Check sheet for the modelled part. Datum: model origin and axes. Units: mm. Give positions to 0.01 mm unless a question says otherwise; leave off trailing zeros. Write each loop counter-clockwise with the first axis right and the second up, starting at its lowest first coordinate (ties: lowest second). Pieces come first, ordered by that corner, then holes. Notation, with made-up numbers: (75.5, -11) -> (116.5, -11) arc R13 cw to (116.5, 5) -> close; hole circle Ø11 at (-29, 58). An arc over 180 degrees is marked (long way). Answer as a JSON object with one key per item and string values.
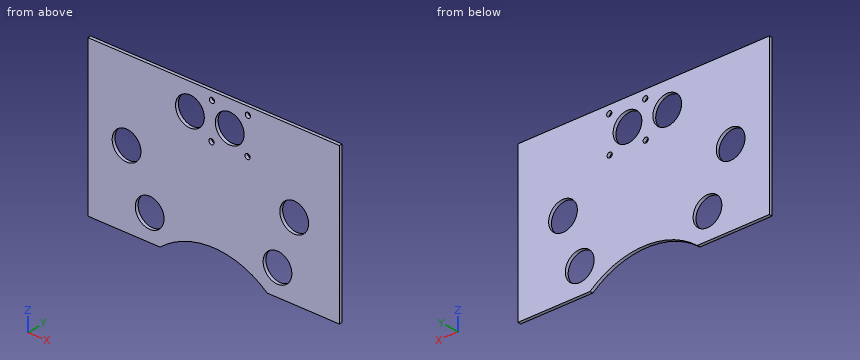
from build123d import *

# Parameters (mm, degrees)
BOSS_EXTRUDE1_DEPTH     = 3.175
F_1_1_115_DOWEL_HOLE1_D = 28.321
F_10_CLEARANCE_HOLE1_D  = 5.1054
F_1_1_115_DOWEL_HOLE3_D = 28.321
SKETCH11_R              = 14.1605
CUT_EXTRUDE1_DEPTH      = 158.031276025
SKETCH12_R              = 14.1605
CUT_EXTRUDE2_DEPTH      = 158.031276025


with BuildPart() as part:
    # Sketch1 → Boss-Extrude1 (new body)
    with BuildSketch(Plane(origin=(0, 0, 0), x_dir=(1, 0, 0), z_dir=(0, 1, 0))):
        with BuildLine():
            Line((-123.825, -55.88), (123.825, -55.88))
            Line((123.825, -55.88), (123.825, 96.52))
            Line((123.825, 96.52), (52.74706153, 96.52))
            ThreePointArc((52.74706153, 96.52), (0, 77.47), (-52.74706153, 96.52))
            Line((-52.74706153, 96.52), (-123.825, 96.52))
            Line((-123.825, 96.52), (-123.825, -55.88))
        make_face()
    extrude(amount=BOSS_EXTRUDE1_DEPTH)

    # 1 (1.115) Dowel Hole1 (through all)
    with Locations(Plane(origin=(0, 3.175, 0), x_dir=(1, 0, 0), z_dir=(0, 1, 0))):
        with Locations((15.875, -30.256942448)):
            Hole(F_1_1_115_DOWEL_HOLE1_D / 2)

    # #10 Clearance Hole1 (through all)
    with Locations(Plane(origin=(0, 3.175, 0), x_dir=(1, 0, 0), z_dir=(0, 1, 0))):
        with Locations((-1.625, -47.756942448), (33.375, -12.756942448), (-2.085512242, -12.296430205), (33.835512242, -48.21745469)):
            Hole(F_10_CLEARANCE_HOLE1_D / 2)

    # 1 (1.115) Dowel Hole3 (through all)
    with Locations(Plane(origin=(-3.175, -34.925, 0), x_dir=(-1, 0, 0), z_dir=(0, -1, 0))):
        with Locations((82.55, 22.098), (-82.55, 22.098)):
            Hole(F_1_1_115_DOWEL_HOLE3_D / 2)

    # Sketch11 → Cut-Extrude1 (cut, through all)
    with BuildSketch(Plane(origin=(0, 3.175, 0), x_dir=(1, 0, 0), z_dir=(0, 1, 0))):
        with Locations(Location((-23.3045, -30.256942448, 0), (0, 0, 270))):
            Circle(SKETCH11_R)
    extrude(amount=-CUT_EXTRUDE1_DEPTH, mode=Mode.SUBTRACT)

    # Sketch12 → Cut-Extrude2 (cut, through all)
    with BuildSketch(Plane(origin=(0, 3.175, 0), x_dir=(1, 0, 0), z_dir=(0, 1, 0))):
        with Locations(Location((-62.933495539, 71.035024331, 0), (0, 0, 270))):
            Circle(SKETCH12_R)
    cut_extrude2 = extrude(amount=-CUT_EXTRUDE2_DEPTH, mode=Mode.SUBTRACT)

    # Mirror2: Cut-Extrude2 across plane
    add(cut_extrude2.mirror(Plane(origin=(0, 0, 0), x_dir=(0, 0, 1), z_dir=(1, 0, 0))), mode=Mode.SUBTRACT)


solid = part.part
1. Sectioned sample at D-D, the plane x = 19. Enter the section's corners in (y, z) (3 decimals), plus the area to 3 significant figures.
Determined:
{"outline": "(0, -79.686) -> (3.175, -79.686) -> (3.175, 16.446) -> (0, 16.446) -> close; (0, 44.068) -> (3.175, 44.068) -> (3.175, 55.88) -> (0, 55.88) -> close", "area": "343 mm^2"}
2. Sectioned sample at A-A, the plane z = -30.5. Enter the section's corners in (x, y) (3 decimals), plus the area to 3 significant figures.
Determined:
{"outline": "(-123.825, 0) -> (-97.124, 0) -> (-97.124, 3.175) -> (-123.825, 3.175) -> close; (-74.326, 0) -> (67.976, 0) -> (67.976, 3.175) -> (-74.326, 3.175) -> close; (90.774, 0) -> (123.825, 0) -> (123.825, 3.175) -> (90.774, 3.175) -> close", "area": "642 mm^2"}
3. Scan lines: L1, parallel to X at y = 1.45, z = -76 (3 decimals); L2, parallel to X at y = 0.75, z = 19.5 (3 decimals); L3, parallel to Z at x = -94.5, y = 2.5. Record each from-to range of solid material in increasing order. Write a range as [from, to].
Determined:
{"L1": "[-123.825, -76.195], [-49.672, 49.672], [76.195, 123.825]", "L2": "[-123.825, -32.514], [-14.095, 6.666], [25.084, 123.825]", "L3": "[-96.52, -33.21], [-10.98, 55.88]"}
4. Sectioned sample at B-B, the plane x = 73. Enter the section's corners in (y, z) (3 decimals).
Determined:
{"outline": "(0, -96.52) -> (3.175, -96.52) -> (3.175, -80.994) -> (0, -80.994) -> close; (0, -61.076) -> (3.175, -61.076) -> (3.175, -34.742) -> (0, -34.742) -> close; (0, -9.454) -> (3.175, -9.454) -> (3.175, 55.88) -> (0, 55.88) -> close"}
5. Sectioned sample at C-C, the plane y = 1.3. State how many separate pieces and enclosed holes the cut face has, plus the area to 3 significant figures.
Determined:
{"separate pieces": "1", "enclosed holes": "10", "area": "32,500 mm^2"}
6. Go/stop test with a flat-tipped pin: P1, Ø22.5, axis at x = 62.93, z = -71.04, coming from the +Y side. Record where the tip stops, or that it passes through.
Determined:
{"P1": "through"}
